Geometry check sheet. Reference: the model listing, model coordinates, mm. Round coordinates to 2 decimals unless told otherwise and drop trailing zeros. Loops run counter-clockwise (first coordinate to the right, second up) from the corner with the lowest first, then second, coordinate; pieces in that order, holes last. Notation, with made-up numbers: (66, -22.5) - (70, -22.5) arc R26 cw to (70, 9.5) - close; hole circle Ø5 at (-2, 83.5). An arc over 180 degrees is marked (long way). Answer as CSV lines item,"result". Start each with the question number.
1) Thickness scan on line 1 along X through (y, z) = (7.75, 5.75) (3 decimals); line 2 along X through (y, z) = (7.25, 4.75) (3 decimals); line 3 along Y through (x, z) = (25, 1.5) (3 decimals). Record the ranges inside material, lowest first.
2) Depth check by flat-ended pin: P1, Ø3, axis at x = 23.81, y = 7.94, coming from the -Z side. Enter the tip coordinate at first touch or a pass-through.
3) Cross-section at A-A on x = 24.5. Record the boundary of the cut face in (y, z) (1 decimal).
4) Cross-section at B-B on y = 7. Record the boundary of the cut face in (x, z) (1 decimal), and give its area (3 significant figures).
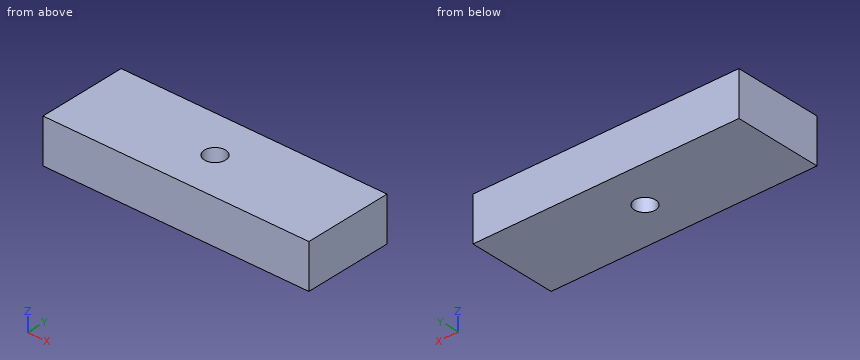
from build123d import *

# Parameters (mm, degrees)
SKETCH1_W                 = 47.625
SKETCH1_H                 = 15.875
BOSS_EXTRUDE1_DEPTH       = 7.9375
F_6_CLEARANCE_HOLE1_D     = 3.7973
F_6_CLEARANCE_HOLE1_DEPTH = 7.9375


with BuildPart() as part:
    # Sketch1 → Boss-Extrude1 (new body)
    with BuildSketch(Plane.XY):
        with Locations((23.8125, 7.9375)):
            Rectangle(SKETCH1_W, SKETCH1_H)
    extrude(amount=BOSS_EXTRUDE1_DEPTH)

    # #6 Clearance Hole1
    with Locations(Plane.XY.offset(7.9375)):
        with Locations((23.8125, 7.9375)):
            Hole(F_6_CLEARANCE_HOLE1_D / 2, depth=F_6_CLEARANCE_HOLE1_DEPTH)


solid = part.part
Answer block:
1,line 1,"x = 0 to 21.923, 25.702 to 47.625"
1,line 2,"x = 0 to 22.043, 25.582 to 47.625"
1,line 3,"y = 0 to 6.456, 9.419 to 15.875"
2,P1,"passes through"
3,outline,"(0, 0) - (6.2, 0) - (6.2, 7.9) - (0, 7.9) - close; (9.7, 0) - (15.9, 0) - (15.9, 7.9) - (9.7, 7.9) - close"
4,outline,"(0, 0) - (22.2, 0) - (22.2, 7.9) - (0, 7.9) - close; (25.5, 0) - (47.6, 0) - (47.6, 7.9) - (25.5, 7.9) - close"
4,area,"352 mm^2"
